```python
from build123d import *

# Parameters (mm, degrees)
F0_R     = 69.360533
F1_DEPTH = 101.6


with BuildPart() as f1:
    # F0 (on Front) → F1 (new body)
    with BuildSketch(Plane.XZ):
        Circle(F0_R)
        Polygon((-31.735938, 57.054307), (33.54251, 56.011282), (65.278448, -1.043025), (31.735938, -57.054307), (-33.54251, -56.011282), (-65.278448, 1.043025), align=None, mode=Mode.SUBTRACT)
    extrude(amount=-F1_DEPTH)


solid = f1.part
```
Read the model definition and answer for the solid it produces. Units are mm, in the model's axes. A direction names the side the tool comes from. Round coordinates to 2 decimals unless told otherwise and drop trailing zeros. Loops run counter-clockwise (first coordinate to the right, second up) from the corner with the lowest first, then second, coordinate; pieces in that order, holes last. Notation, with made-up numbers: (-9, 88.25) -> (12, 88.25) arc R28 ccw to (12, 118.25) -> close; hole circle Ø2 at (-4.5, 81.25). An arc over 180 degrees is marked (long way). One line per item, written item: value.
1) A cutting plane is placed at A-A (y = 45). Determine the outline of the cut face in (x, z).
Answer list:
outline: circle Ø138.72 at (0, 0); hole (-65.28, 1.04) -> (-33.54, -56.01) -> (31.74, -57.05) -> (65.28, -1.04) -> (33.54, 56.01) -> (-31.74, 57.05) -> close
2) Consider L1, parallel to X at y = 47, z = 40; L2, parallel to Z at x = 4, y = 62; L3, parallel to Z at x = 55.5, y = 79.5. Determine where each line is inside the solid, lowest interval first. Write a range as [from, to].
Answer list:
L1: x = [-56.66, -41.95], [42.45, 56.66]
L2: z = [-69.25, -56.61], [56.48, 69.25]
L3: z = [-41.6, -17.37], [16.54, 41.6]
3) For faces 4 (the face through (0, 101.6, 57)), 5 (the face through (48.74, 50.09, -28.66)), determine the directions among +Z, -Z, +X, -X, +Y, -Y from which every point of the face is accessible in a straight line to the end or side of a thin tool.
Answer list:
face 4: +Z, -Z, +X, -X, +Y
face 5: +Y, -Y
4) A cutting plane is placed at C-C (z = 27). Determine the outline of the cut face in (x, y).
Answer list:
outline: (-63.89, 0) -> (-49.73, 0) -> (-49.73, 101.6) -> (-63.89, 101.6) -> close; (49.68, 0) -> (63.89, 0) -> (63.89, 101.6) -> (49.68, 101.6) -> close
5) Flat-ended cylindrical pins translate along their axes: P1, Ø1.5, axis at x = 38.5, y = 10.5, coming from the -Z side; P2, Ø10, axis at x = -32.5, y = 69.5, coming from the +Z side; P3, Ø2, axis at y = 61.5, z = -52, coming from the +X side. Find the tip coordinate at first contact, or state that the pin passes through.
Answer list:
P1: stops at z = -58.19
P2: stops at z = 63.68
P3: stops at x = 47.01
6) The mould has two halves that part along Z. Classify faces 1 (the face through (49.19, 50.09, 27.88)), 2 (the face through (-55.042, 50.089, -42.205)), 3 (the face through (0, 0, 57)): pulls with the +Z half, pulls with the -Z half, needs draft (parallel to the pull), parting line crosses it, or undercut.
Answer list:
face 1: undercut
face 2: parting line crosses it
face 3: needs draft
7) A cutting plane is placed at B-B (x = 0). Determine the outline of the cut face in (y, z), and give its area (3 significant figures).
Answer list:
outline: (0, -69.36) -> (101.6, -69.36) -> (101.6, -56.55) -> (0, -56.55) -> close; (0, 56.55) -> (101.6, 56.55) -> (101.6, 69.36) -> (0, 69.36) -> close
area: 2,600 mm²
